CAD build for the part. Positions are in the model's coordinates, mm. Give positions to 0.01 mm unless a question says otherwise; leave off trailing zeros. Write each loop counter-clockwise with the first axis right and the second up, starting at its lowest first coordinate (ties: lowest second). Pieces come first, ordered by that corner, then holes. Notation, with made-up numbers: (61.25, -40) - (95.25, -40) arc R21 ccw to (95.25, -7) - close; hole circle Ø3 at (11.25, 53). An arc over 180 degrees is marked (long way). Answer as a JSON object with one key per item and string values.
from build123d import *

# Parameters (mm, degrees)
SKETCH1_R           = 23.241
BOSS_EXTRUDE1_DEPTH = 12.192


with BuildPart() as part:
    # Sketch1 → Boss-Extrude1 (new body)
    with BuildSketch(Plane.XY):
        with BuildLine():
            Line((-44.45, 76.2), (44.45, 76.2))
            ThreePointArc((44.45, 76.2), (48.940128061, 74.340128061), (50.8, 69.85))
            Line((50.8, 69.85), (50.8, -69.85))
            Line((50.8, -69.85), (50.8, -120.65))
            Line((50.8, -120.65), (-50.8, -120.65))
            Line((-50.8, -120.65), (-50.8, -69.85))
            Line((-50.8, -69.85), (-50.8, 69.85))
            ThreePointArc((-50.8, 69.85), (-48.940128061, 74.340128061), (-44.45, 76.2))
        make_face()
        with Locations((0, 29.718)):
            Circle(SKETCH1_R, mode=Mode.SUBTRACT)
        with Locations((0, -29.718)):
            Circle(SKETCH1_R, mode=Mode.SUBTRACT)
    extrude(amount=-BOSS_EXTRUDE1_DEPTH)


solid = part.part
Item 1: Cut at D-D (y = 26). Give the cut face in (x, z).
Entries:
{"outline": "(-50.8, -12.19) - (-22.94, -12.19) - (-22.94, 0) - (-50.8, 0) - close; (22.94, -12.19) - (50.8, -12.19) - (50.8, 0) - (22.94, 0) - close"}
Item 2: Probe line 1 (Y direction, x = 1, z = -6); line 2 (Y direction, x = 0, z = -7); line 3 (X direction, y = -30.5, z = -11.5). List the from-to ranges inside material, lowest first. Write a range as from..to.
Entries:
{"line 1": "-120.65..-52.94, -6.5..6.5, 52.94..76.2", "line 2": "-120.65..-52.96, -6.48..6.48, 52.96..76.2", "line 3": "-50.8..-23.23, 23.23..50.8"}
Item 3: Cut at A-A (x = 0). Give the cut face in (y, z), and give its area (3 significant figures).
Entries:
{"outline": "(-120.65, -12.19) - (-52.96, -12.19) - (-52.96, 0) - (-120.65, 0) - close; (-6.48, -12.19) - (6.48, -12.19) - (6.48, 0) - (-6.48, 0) - close; (52.96, -12.19) - (76.2, -12.19) - (76.2, 0) - (52.96, 0) - close", "area": "1,270 mm2"}
Item 4: Mould opens along X. For faces 1 (the cylindrical face through (48.89, 74.39, -6.01)), 2 (the cylindrical face through (-48.99, 74.29, -6.01)), 3 (the cylindrical face through (12.49, -10.12, -6.01)) say: +X half, -X half, draft (parallel to the pull), parting line (faces both ways), or undercut.
Entries:
{"face 1": "+X half", "face 2": "-X half", "face 3": "undercut"}
Item 5: Cut at C-C (z = -9.25). Give the cut face in (x, y), and give its area (3 significant figures).
Entries:
{"outline": "(-50.8, -120.65) - (50.8, -120.65) - (50.8, 69.85) arc R6.35 ccw to (44.45, 76.2) - (-44.45, 76.2) arc R6.35 ccw to (-50.8, 69.85) - close; hole circle Ø46.48 at (0, -29.72); hole circle Ø46.48 at (0, 29.72)", "area": "16,600 mm2"}
Item 6: Cut at B-B (y = 46.5). Give the cut face in (x, z).
Entries:
{"outline": "(-50.8, -12.19) - (-16.08, -12.19) - (-16.08, 0) - (-50.8, 0) - close; (16.08, -12.19) - (50.8, -12.19) - (50.8, 0) - (16.08, 0) - close"}
